Study the drawing (mm; zero at the part's minimum x, y, z) and answer. Give positions to 0.01 mm unless a question says otherwise; leave off trailing zeros. Order: outer loops, then holes, each group sorted by start corner. A loop starts at its lowest first (then second) coordinate and runs counter-clockwise, first axis right, second up. Notation, with made-up numbers: (47, 42.25) - (96, 42.25) arc R22 cw to (96, 49.25) - close; hole circle Ø5 at (-33, 24). An arc over 180 degrees is marked (long way). Put each result on its own line as item: value.
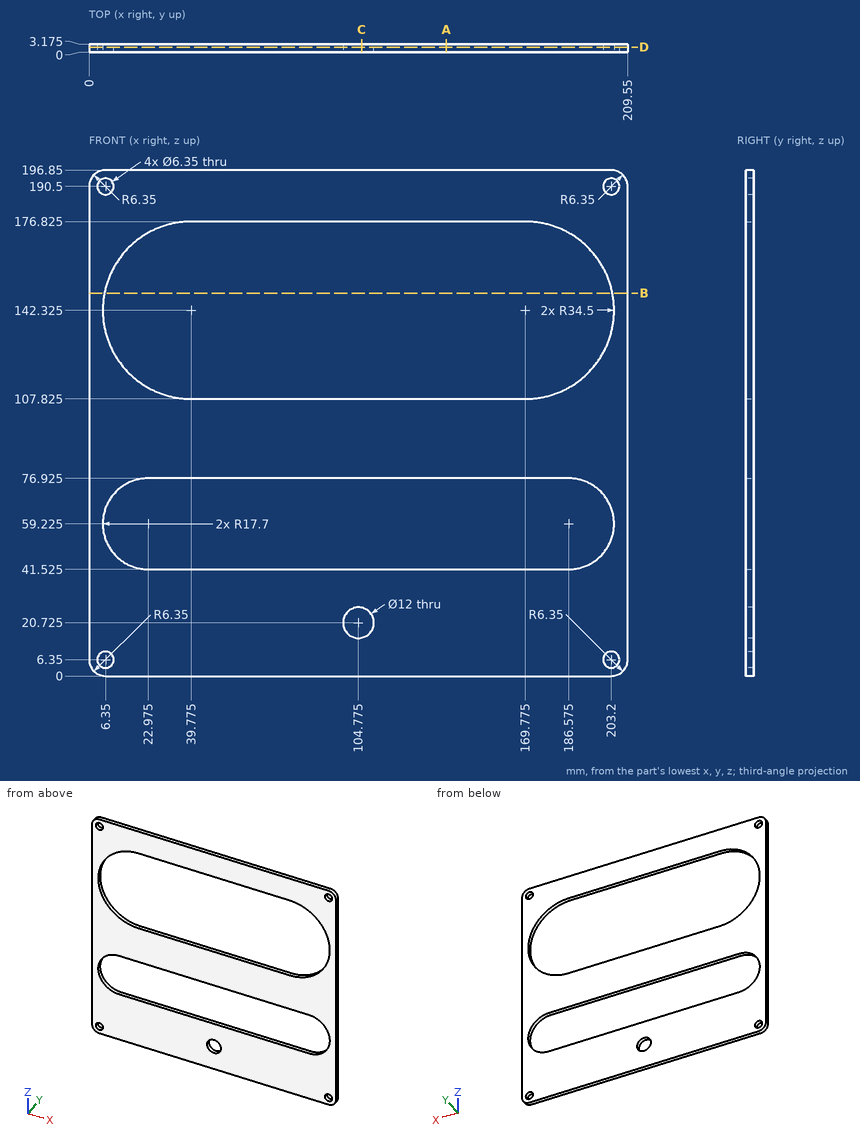
(1) Straight lines are drawn through the part: line 1 (Z direction, x = 114, y = 2.45) (3 decimals); line 2 (X direction, y = 0.6, z = 58.5); line 3 (Z direction, x = 185.5, y = 3) (3 decimals). For each, find the intervals that lie inside material, in ascending order.
Geometry check:
line 1: z = 0 to 41.525, 76.925 to 107.825, 176.825 to 196.85
line 2: x = 0 to 5.29, 204.26 to 209.55
line 3: z = 0 to 41.525, 76.925 to 111.617, 173.033 to 196.85
(2) Section B-B, the plane z = 149 is taken. Write down the section's boundary in (x, y) (3 decimals).
Geometry check:
outline: (0, 0) - (5.927, 0) - (5.927, 3.175) - (0, 3.175) - close; (203.623, 0) - (209.55, 0) - (209.55, 3.175) - (203.623, 3.175) - close
(3) Section C-C, the plane x = 106 is taken. Write down the section's boundary in (y, z) (3 decimals).
Geometry check:
outline: (0, 0) - (3.175, 0) - (3.175, 14.851) - (0, 14.851) - close; (0, 26.599) - (3.175, 26.599) - (3.175, 41.525) - (0, 41.525) - close; (0, 76.925) - (3.175, 76.925) - (3.175, 107.825) - (0, 107.825) - close; (0, 176.825) - (3.175, 176.825) - (3.175, 196.85) - (0, 196.85) - close
(4) Section D-D, the plane y = 2 is taken. Write down the section's boundary in (x, z) (3 decimals).
Geometry check:
outline: (0, 6.35) arc R6.35 ccw to (6.35, 0) - (203.2, 0) arc R6.35 ccw to (209.55, 6.35) - (209.55, 190.5) arc R6.35 ccw to (203.2, 196.85) - (6.35, 196.85) arc R6.35 ccw to (0, 190.5) - close; hole circle Ø6.35 at (6.35, 6.35); hole circle Ø6.35 at (6.35, 190.5); hole (22.975, 41.525) - (186.575, 41.525) arc R17.7 ccw to (186.575, 76.925) - (22.975, 76.925) arc R17.7 ccw to start; hole (39.775, 107.825) - (169.775, 107.825) arc R34.5 ccw to (169.775, 176.825) - (39.775, 176.825) arc R34.5 ccw to start; hole circle Ø12 at (104.775, 20.725); hole circle Ø6.35 at (203.2, 6.35); hole circle Ø6.35 at (203.2, 190.5)
(5) Section A-A, the plane x = 139 is taken. Write down the section's boundary in (y, z) (3 decimals).
Geometry check:
outline: (0, 0) - (3.175, 0) - (3.175, 41.525) - (0, 41.525) - close; (0, 76.925) - (3.175, 76.925) - (3.175, 107.825) - (0, 107.825) - close; (0, 176.825) - (3.175, 176.825) - (3.175, 196.85) - (0, 196.85) - close
